Verification items for the finished model (mm, model axes). Face numbers are marked on the shaded views. A direction names the side the tool comes from. Give positions to 0.01 mm unless a question says otherwise; leave off trailing zeros. Order: outer loops, then holes, each group sorted by start corner. A loop starts at its lowest first (then second) coordinate and runs counter-clockwise, first axis right, second up. Notation, with made-up numbers: (26.25, 46.25) -> (36.25, 46.25) arc R22 cw to (36.25, 74.25) -> close; hole circle Ø6 at (23, -27). An arc over 180 degrees is marked (long way). Return JSON: item names as keys, results as strings. Group by question number.
(1) Thickness scan on line 1 along X through (y, z) = (-35, 10); line 2 along Y through (x, z) = (-125, 7); line 3 along X through (y, z) = (10, 15.25). Record the ranges inside material, lowest first.
(2) Depth check by flat-ended pin: pin 1 Ø1 at (x, z) = (126.5, 5.5) entering from +Y; pin 2 Ø5 at (x, z) = (-31.5, 10.5) entering from +Y; pin 3 Ø10 at (x, z) = (-65, 10) entering from -Y. Enter the tip coordinate at first touch or a pass-through.
(3) Tool access check on the marked faces 1 and 2. Record the directions out of +Z, -Z, +X, -X, +Y, -Y that give a thin tool (end or side, any length) a straight path to the whole face; none if there is none.
(4) Cross-section at B-B on x = 125. Enter the section's corners in (y, z).
(5) Cross-section at C-C on y = -55.5. Enter the section's corners in (x, z).
(6) Cross-section at A-A on z = 10. Enter the section's corners in (x, y), then the cut area to 3 significant figures.
(7) Cross-section at D-D on x = 0. Enter the section's corners in (y, z).
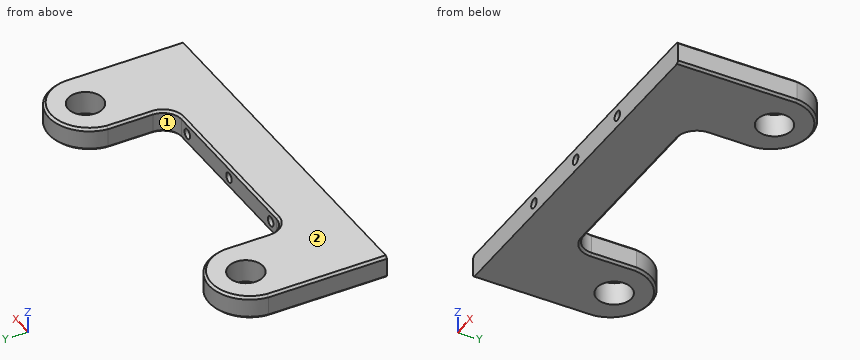
Autodesk Fusion 360 part; units mm, degrees
sketch "Sketch1" plane through (0, 0, 0) normal (0, 0, 1) x (1, 0, 0)
  line L0 (160, -67.5) -> (-160, -67.5)
  line L1 (-160, -67.5) -> (-160, 67.5)
  line L2 (-160, 67.5) -> (160, 67.5)
  line L3 (160, 67.5) -> (160, -67.5)
  line L4 (160, -67.5) -> (-160, 67.5) construction
  line L5 (-160, -67.5) -> (160, 67.5) construction
  line L6 (-160, 67.5) -> (-125, 67.5)
  line L7 (-125, 67.5) -> (-125, 42.5)
  line L8 (-125, 42.5) -> (-160, 42.5)
  line L9 (-160, 42.5) -> (-160, 67.5)
  line L10 (125, 42.5) -> (160, 42.5)
  line L11 (160, 42.5) -> (160, 67.5)
  line L12 (160, 67.5) -> (125, 67.5)
  line L13 (125, 67.5) -> (125, 42.5)
  dimension "d1" = 320
  dimension "d2" = 135
  dimension "d3" = 35
  dimension "d4" = 35
  dimension "d5" = 25
  dimension "d6" = 25
extrude "Extrude1" add sketch "Sketch1" along normal blind 20
sketch "Sketch2" plane through (0, 0, 20) normal (0, 0, 1) x (1, 0, 0)
  line L0 (160, -67.5) -> (160, 67.5)
  line L1 (160, 67.5) -> (-160, 67.5)
  line L2 (-160, 67.5) -> (-160, -67.5)
  line L3 (-160, -67.5) -> (160, -67.5)
  line L4 (-125, 35.633) -> (125, 35.633)
  dimension "d9" = 250
  dimension "d11" = 103.133
hole "Hole1" at (-125, 35.633, 20) at (125, 35.633, 20) direction (0, 0, -1) diameter 30 depth 50 tip angle 118
sketch "Sketch3" plane through (0, 0, 20) normal (0, 0, 1) x (1, 0, 0)
  circle A0 centre (-125, 35.633) radius 15
  circle A1 centre (125, 35.633) radius 15
  line L0 (160, -67.5) -> (160, 67.5)
  line L1 (160, 67.5) -> (-160, 67.5)
  line L2 (-160, 67.5) -> (-160, -67.5)
  line L3 (-160, -67.5) -> (160, -67.5)
  line L4 (-125, 35.633) -> (-160, 35.633)
  line L5 (125, 35.633) -> (126.752, 35.633)
  line L6 (126.752, 35.633) -> (160, 35.633)
  line L7 (125, 35.633) -> (90, 35.633)
  line L8 (-125, 35.633) -> (-90, 35.633)
  line L9 (-90, 35.633) -> (-90, -19.367)
  line L10 (90, 35.633) -> (90, -19.367)
  line L11 (-90, -19.367) -> (90, -19.367)
  line L12 (-125, 35.633) -> (-125, 67.5)
  line L13 (125, 35.633) -> (125, 67.5)
  arc A2 (-90, 35.633) -> (-160, 35.633) centre (-125, 32.346) ccw
  arc A3 (160, 35.633) -> (90, 35.633) centre (125, 32.346) ccw
  dimension "d15" = 55
  dimension "d16" = 70
  dimension "d17" = 55
extrude "Extrude2" cut sketch "Sketch3" against normal blind 20 contours L1 L9 L10 L11 A2 A3 | L1 L2 A2 | L0 L1 A3
sketch "Sketch4" plane through (0, -19.367, 0) normal (0, 1, 0) x (-1, 0, 0)
  line L0 (90, 20) -> (-90, 20)
  line L1 (-90, 20) -> (-90, 0)
  line L2 (-90, 0) -> (90, 0)
  line L3 (90, 0) -> (90, 20)
  line L4 (90, 10) -> (65, 10)
  line L5 (-90, 10) -> (-65, 10)
  line L6 (0, 10) -> (-25, 10)
  dimension "d20" = 25
  dimension "d21" = 25
  dimension "d22" = 10
  dimension "d23" = 10
  dimension "d24" = 25
  dimension "d25" = 10
hole "Hole2" at (-65, -19.367, 10) at (0, -19.367, 10) at (65, -19.367, 10) direction (0, -1, 0) diameter 8.5 end through all
fillet "Fillet1" radius 16 2 edges at (-90, -19.367, 10) (90, -19.367, 10)
chamfer "Chamfer1" distance 2 angle 45 18 edges at (-125, 67.5, 20) (-90, 16.133, 20) (90, 16.133, 20) (85.3137, -14.6807, 20) (0, -19.367, 20) (-85.3137, -14.6807, 20) (125, 67.5, 20) (160, -15.9335, 20) (-160, -15.9335, 20) (160, -15.9335, 0) (125, 67.5, 0) (90, 16.133, 0) (-90, 16.133, 0) (-85.3137, -14.6807, 0) (0, -19.367, 0) (85.3137, -14.6807, 0) (-125, 67.5, 0) (-160, -15.9335, 0)
equation "d2 = 160 mm - 25 mm"
equation "d9 = 320 mm - 35 mm - 35 mm"
equation "d11 = 88.133 mm + 15 mm"
Verdict:
{
 "1": {"line 1": "-160 to -69.25, -60.75 to -4.25, 4.25 to 60.75, 69.25 to 160", "line 2": "-67.5 to 20.63, 50.63 to 67.5", "line 3": "-160 to -90, 90 to 160"},
 "2": {"pin 1": "y = 67.49", "pin 2": "y = -19.37", "pin 3": "y = -67.5"},
 "3": {"face 1": "+Z, -Z, +Y", "face 2": "+Z, +X, -X, +Y, -Y"},
 "4": {"outline": "(-67.5, 0) -> (20.63, 0) -> (20.63, 20) -> (-67.5, 20) -> close; (50.63, 0) -> (65.5, 0) -> (67.5, 2) -> (67.5, 18) -> (65.5, 20) -> (50.63, 20) -> close"},
 "5": {"outline": "(-160, 2) -> (-158, 0) -> (158, 0) -> (160, 2) -> (160, 18) -> (158, 20) -> (-158, 20) -> (-160, 18) -> close; hole circle Ø8.5 at (-65, 10); hole circle Ø8.5 at (0, 10); hole circle Ø8.5 at (65, 10)"},
 "6": {"outline": "(-160, -67.5) -> (-69.25, -67.5) -> (-69.25, -19.37) -> (-74, -19.37) arc R16 cw to (-90, -3.37) -> (-90, 35.63) arc R35.15 ccw to (-160, 35.63) -> close; (-60.75, -67.5) -> (-4.25, -67.5) -> (-4.25, -19.37) -> (-60.75, -19.37) -> close; (4.25, -67.5) -> (60.75, -67.5) -> (60.75, -19.37) -> (4.25, -19.37) -> close; (69.25, -67.5) -> (160, -67.5) -> (160, 35.63) arc R35.15 ccw to (90, 35.63) -> (90, -3.37) arc R16 cw to (74, -19.37) -> (69.25, -19.37) -> close; hole circle Ø30 at (-125, 35.63); hole circle Ø30 at (125, 35.63)", "area": "24,000 mm²"},
 "7": {"outline": "(-67.5, 0) -> (-21.37, 0) -> (-19.37, 2) -> (-19.37, 5.75) -> (-67.5, 5.75) -> close; (-67.5, 14.25) -> (-19.37, 14.25) -> (-19.37, 18) -> (-21.37, 20) -> (-67.5, 20) -> close"}
}
